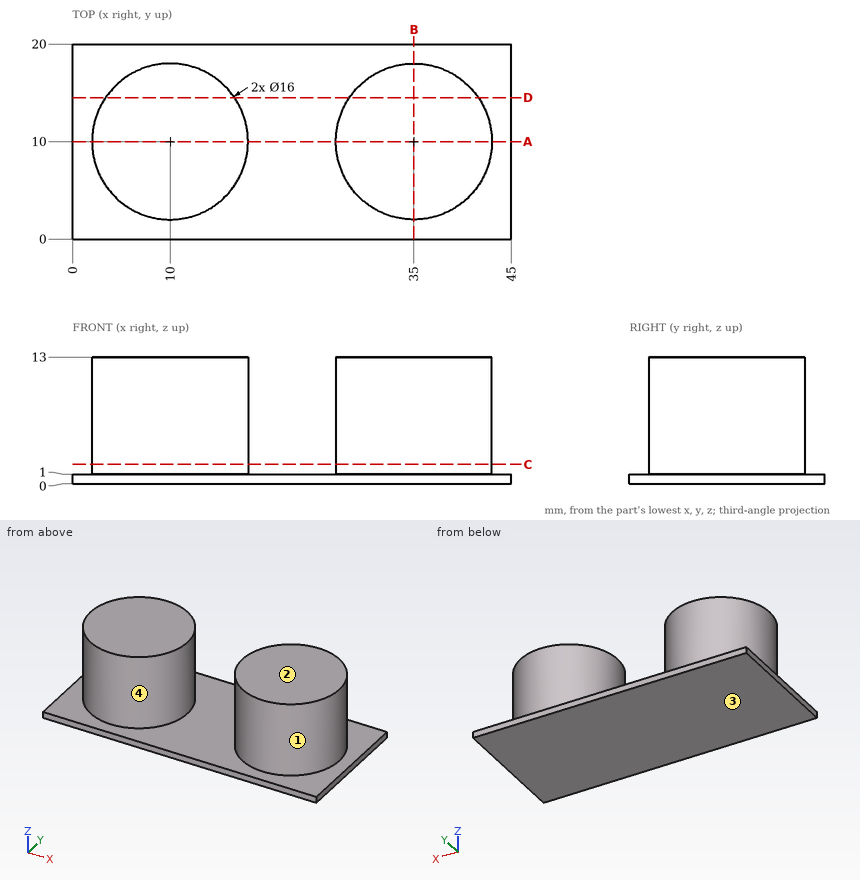
The figure shows three views and two pictorial views of one solid part (mm, origin at its lowest corner). Answer the questions. A direction names the side the tool comes from. Coordinates: 2 decimals unless noted, no trailing zeros. Loops run counter-clockwise (first coordinate to the right, second up) from the corner with the lowest first, then second, coordinate; pieces in that order, holes last. Notation, with made-up numbers: (28, -35.5) - (33, -35.5) arc R18 ccw to (33, -24.5) - close; hole circle Ø7 at (-34, 4.25). An arc over 180 degrees is marked (long way). Answer in a Markdown table with one row per item.
Q1. For the marked faces 1 and 2, determine the directions among +Z, -Z, +X, -X, +Y, -Y from which every point of the face is accessible in a straight line to the end or side of a thin tool.
Here are the results:
| item | result |
|---|---|
| face 1 | +Z |
| face 2 | +Z, +X, -X, +Y, -Y |
Q2. Find section A-A on y = 10. Write down the section's boundary in (x, z), plus the area to 3 significant figures.
Here are the results:
| item | result |
|---|---|
| outline | (0, 0) - (45, 0) - (45, 1) - (43, 1) - (43, 13) - (27, 13) - (27, 1) - (18, 1) - (18, 13) - (2, 13) - (2, 1) - (0, 1) - close |
| area | 429 mm^2 |
Q3. The mould has two halves that part along X. Classify the marked faces 3 and 4: pulls with the +X half, pulls with the -X half, needs draft (parallel to the pull), parting line crosses it, or undercut.
Here are the results:
| item | result |
|---|---|
| face 3 | needs draft |
| face 4 | undercut |
Q4. Find section D-D on y = 14.5. Write down the section's boundary in (x, z), plus the area to 3 significant figures.
Here are the results:
| item | result |
|---|---|
| outline | (0, 0) - (45, 0) - (45, 1) - (41.61, 1) - (41.61, 13) - (28.39, 13) - (28.39, 1) - (16.61, 1) - (16.61, 13) - (3.39, 13) - (3.39, 1) - (0, 1) - close |
| area | 362 mm^2 |
Q5. Find section C-C on z = 2. Write down the section's boundary in (x, y).
Here are the results:
| item | result |
|---|---|
| outline | circle Ø16 at (10, 10); circle Ø16 at (35, 10) |
Q6. Given P1, Ø3, axis at y = 14, z = 8.5, coming from the -X side; P2, Ø1.5, axis at x = 21.5, z = 2, coming from the -Y side; P3, Ø6, axis at x = 22.5, y = 11.5, coming from the +Z side; P4, Ø1, axis at x = 13, z = 8, coming from the +Y side, each flat-ended and moving along its own axis, determine where each tip first touches the part or whether it passes through.
Here are the results:
| item | result |
|---|---|
| P1 | stops at x = 2.4 |
| P2 | passes through |
| P3 | stops at z = 1 |
| P4 | stops at y = 17.6 |
Q7. Straight lines are drawn through the part: line 1 along Z through (x, y) = (26, 3.25); line 2 along X through (y, z) = (8.75, 1.25); line 3 along X through (y, z) = (16.25, 7.25). For each, find the intervals that lie inside material, in ascending order. Write a range as [from, to].
Here are the results:
| item | result |
|---|---|
| line 1 | z = [0, 1] |
| line 2 | x = [2.1, 17.9], [27.1, 42.9] |
| line 3 | x = [5.01, 14.99], [30.01, 39.99] |
Q8. Find section B-B on x = 35. Write down the section's boundary in (y, z), plus the area to 3 significant figures.
Here are the results:
| item | result |
|---|---|
| outline | (0, 0) - (20, 0) - (20, 1) - (18, 1) - (18, 13) - (2, 13) - (2, 1) - (0, 1) - close |
| area | 212 mm^2 |
